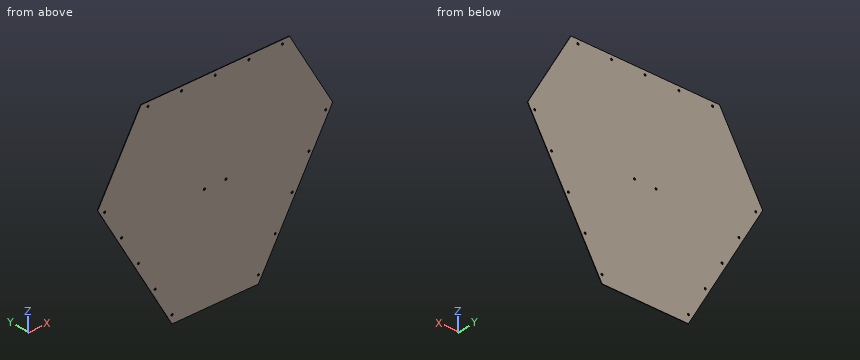
Autodesk Inventor part; units mm, degrees
ref_plane "YZ Plane" through (0, 0, 0) normal (1, 0, 0) x (0, 1, 0)
ref_plane "XZ Plane" through (0, 0, 0) normal (0, 1, 0) x (-1, 0, 0)
ref_plane "XY Plane" through (0, 0, 0) normal (0, 0, 1) x (1, 0, 0)
sketch "Sketch1" plane through (0, 0, 0) normal (0, 1, 0) x (-1, 0, 0)
  line L0 (101.5, -410.6115) -> (-101.7, -410.6115)
  line L1 (101.5, -410.6115) -> (406.3, 117.3176)
  line L2 (406.3, 117.3176) -> (304.7, 293.2939)
  line L3 (304.7, 293.2939) -> (-304.9, 293.2939)
  line L4 (-304.9, 293.2939) -> (-406.5, 117.3176)
  line L5 (-304.9, 293.2939) -> (-101.7, 293.2939) construction
  line L6 (-406.5, 117.3176) -> (-101.7, -410.6115)
  line L7 (-0.1, -410.6115) -> (-0.1, 293.2939) construction
  line L8 (-355.7, 205.3058) -> (253.9, -146.647) construction
  line L9 (-254.1, -146.647) -> (355.5, 205.3058) construction
  line L10 (34.1394, 19.7104) -> (0, 0) construction
  line L11 (0, 0) -> (-34.1644, -19.6671) construction
  line L12 (0, 0) -> (34.1144, -19.7537) construction
  circle A0 centre (-34.1644, -19.6671) radius 3.175 construction
  circle A1 centre (34.1144, -19.7537) radius 3.175 construction
  dimension "d0" = 120
  dimension "d1" = 203.2
  dimension "d3" = 609.6
  dimension "d8" = 203.2
  dimension "d10" = 120
  dimension "d13" = 609.6
  dimension "d15" = 203.2
  dimension "d16" = 120
  dimension "d17" = 609.6
  dimension "d18" = 120
  dimension "d22" = 101.6
  dimension "d122" = 39.4208
  dimension "d123" = 39.4208
  dimension "d124" = 6.35
  dimension "d125" = 6.35
extrude "Extrusion1" add sketch "Sketch1" against normal blind 1.5
sketch "Sketch2" plane through (0, 0, 0) normal (0, 1, 0) x (1, 0, 0)
  line L0 (-101.5, 410.6115) -> (101.7, 410.6115)
  line L1 (-406.3, -117.3176) -> (-101.5, 410.6115)
  line L2 (-304.7, -293.2939) -> (-406.3, -117.3176)
  line L3 (304.9, -293.2939) -> (-304.7, -293.2939)
  line L4 (406.5, -117.3176) -> (304.9, -293.2939)
  line L5 (101.7, 410.6115) -> (406.5, -117.3176)
  line L6 (0.1, 410.6115) -> (0.1, 350.0579) construction
  line L7 (0.1, 350.0579) -> (136.6606, 350.0579) construction
  line L8 (0.1, 350.0579) -> (-136.4606, 350.0579) construction
  line L9 (-355.5, -205.3058) -> (-303.059, -175.029) construction
  line L10 (355.7, -205.3058) -> (303.259, -175.029) construction
  line L11 (303.259, -175.029) -> (371.5394, -56.764) construction
  line L12 (303.259, -175.029) -> (234.9787, -293.2939) construction
  line L13 (-303.059, -175.029) -> (-234.7787, -293.2939) construction
  line L14 (-303.059, -175.029) -> (-371.3394, -56.764) construction
  line L15 (-371.3394, -56.764) -> (-234.7787, -293.2939)
  line L16 (-304.7, -293.2939) -> (-234.7787, -293.2939)
  line L17 (-304.7, -293.2939) -> (-406.3, -117.3176)
  line L18 (-371.3394, -56.764) -> (-406.3, -117.3176)
  line L19 (-101.5, 410.6115) -> (-136.4606, 350.0579)
  line L20 (-101.5, 410.6115) -> (101.7, 410.6115)
  line L21 (136.6606, 350.0579) -> (101.7, 410.6115)
  line L22 (136.6606, 350.0579) -> (-136.4606, 350.0579)
  line L23 (371.5394, -56.764) -> (234.9787, -293.2939)
  line L24 (304.9, -293.2939) -> (234.9787, -293.2939)
  line L25 (304.9, -293.2939) -> (406.5, -117.3176)
  line L26 (406.5, -117.3176) -> (371.5394, -56.764)
  point P0 (0, 0)
  dimension "d25" = 60.5536
  dimension "d26" = 60.5536
  dimension "d27" = 118.265
  dimension "d28" = 118.265
  dimension "d29" = 118.265
  dimension "d30" = 118.265
  dimension "d31" = 136.5606
  dimension "d32" = 136.5606
extrude "Extrusion2" cut sketch "Sketch2" against normal blind 25.4 contours L0 L5 L22 L1 | L15 L3 L2 L1 | L5 L4 L3 L23
sketch "Sketch5" plane through (0, -1.5, 0) normal (0, -1, 0) x (1, 0, 0)
  line L0 (-234.7787, 293.2939) -> (-371.3394, 56.764)
  line L1 (-136.4606, -350.0579) -> (136.6606, -350.0579)
  line L2 (136.6606, -350.0579) -> (371.5394, 56.764)
  line L3 (371.5394, 56.764) -> (234.9787, 293.2939)
  line L4 (-303.059, 175.029) -> (-281.062, 162.329) construction
  line L5 (303.259, 175.029) -> (281.262, 162.329) construction
  line L6 (0.1, -350.0579) -> (0.1, -324.6579) construction
  line L7 (-371.3394, 56.764) -> (-349.3423, 44.064) construction
  line L8 (234.9787, 293.2939) -> (212.9817, 280.5939) construction
  line L9 (371.5394, 56.764) -> (349.5423, 44.064) construction
  line L10 (-136.4606, -350.0579) -> (-136.4606, -324.6579) construction
  line L11 (136.6606, -350.0579) -> (136.6606, -324.6579) construction
  line L12 (-136.4606, -324.6579) -> (-136.4606, -324.6579) construction
  line L13 (136.6606, -324.6579) -> (136.6606, -324.6579) construction
  line L14 (-349.3423, 44.064) -> (-349.3423, 44.064) construction
  line L15 (-234.7787, 293.2939) -> (-212.7817, 280.5939) construction
  line L16 (-212.7817, 280.5939) -> (-212.7817, 280.5939) construction
  circle A0 centre (-349.3423, 44.064) radius 3.175
  circle A1 centre (-212.7817, 280.5939) radius 3.175
  circle A2 centre (212.9817, 280.5939) radius 3.175
  circle A3 centre (349.5423, 44.064) radius 3.175
  circle A4 centre (136.6606, -324.6579) radius 3.175
  circle A5 centre (-136.4606, -324.6579) radius 3.175
  line L17 (212.9817, 280.5939) -> (212.9817, 280.5939)
  line L18 (349.5423, 44.064) -> (349.5423, 44.064)
  line L19 (-212.7817, 280.5939) -> (-106.3408, 280.5939) construction
  line L20 (-106.3408, 280.5939) -> (0.1, 280.5939) construction
  line L21 (0.1, 280.5939) -> (106.5408, 280.5939) construction
  line L22 (106.5408, 280.5939) -> (212.9817, 280.5939) construction
  circle A6 centre (-106.3408, 280.5939) radius 3.175
  circle A7 centre (0.1, 280.5939) radius 3.175
  circle A8 centre (106.5408, 280.5939) radius 3.175
  line L23 (-349.3423, 44.064) -> (-296.1219, -48.1165) construction
  line L24 (-296.1219, -48.1165) -> (-242.9015, -140.297) construction
  line L25 (-242.9015, -140.297) -> (-189.6811, -232.4774) construction
  line L26 (-189.6811, -232.4774) -> (-136.4606, -324.6579) construction
  circle A9 centre (-296.1219, -48.1165) radius 3.175
  circle A10 centre (-242.9015, -140.297) radius 3.175
  circle A11 centre (-189.6811, -232.4774) radius 3.175
  line L27 (136.6606, -324.6579) -> (189.8811, -232.4774) construction
  line L28 (189.8811, -232.4774) -> (243.1015, -140.297) construction
  line L29 (243.1015, -140.297) -> (296.3219, -48.1165) construction
  line L30 (296.3219, -48.1165) -> (349.5423, 44.064) construction
  circle A12 centre (189.8811, -232.4774) radius 3.175
  circle A13 centre (243.1015, -140.297) radius 3.175
  circle A14 centre (296.3219, -48.1165) radius 3.175
  point P0 (0, 0)
  dimension "d67" = 25.4
  dimension "d68" = 25.4
  dimension "d69" = 25.4
  dimension "d70" = 25.4
  dimension "d71" = 25.4
  dimension "d72" = 25.4
  dimension "d73" = 0
  dimension "d74" = 0
  dimension "d75" = 0
  dimension "d76" = 0
  dimension "d77" = 6.35
  dimension "d78" = 6.35
  dimension "d79" = 6.35
  dimension "d80" = 6.35
  dimension "d81" = 6.35
  dimension "d82" = 6.35
  dimension "d83" = 0
  dimension "d84" = 0
  dimension "d87" = 425.7634
  dimension "d88" = 106.4408
  dimension "d89" = 106.4408
  dimension "d90" = 106.4408
  dimension "d91" = 106.4408
  dimension "d92" = 6.35
  dimension "d93" = 6.35
  dimension "d94" = 6.35
  dimension "d95" = 106.4408
  dimension "d96" = 106.4408
  dimension "d97" = 106.4408
  dimension "d98" = 106.4408
  dimension "d99" = 6.35
  dimension "d100" = 6.35
  dimension "d101" = 6.35
  dimension "d102" = 106.4408
  dimension "d103" = 106.4408
  dimension "d104" = 106.4408
  dimension "d105" = 106.4408
  dimension "d106" = 6.35
  dimension "d107" = 6.35
  dimension "d108" = 6.35
extrude "Extrusion5" cut sketch "Sketch5" against normal blind 25.4 contours A0 | A1 | A2 | A3 | A4 | A5
sketch "Sketch6" plane through (0, -1.5, 0) normal (0, -1, 0) x (1, 0, 0)
  circle A0 centre (-106.3408, 280.5939) radius 3.175
  circle A1 centre (0.1, 280.5939) radius 3.175
  circle A2 centre (106.5408, 280.5939) radius 3.175
  circle A3 centre (-296.1219, -48.1165) radius 3.175
  circle A4 centre (-242.9015, -140.297) radius 3.175
  circle A5 centre (-189.6811, -232.4774) radius 3.175
  circle A6 centre (189.8811, -232.4774) radius 3.175
  circle A7 centre (243.1015, -140.297) radius 3.175
  circle A8 centre (296.3219, -48.1165) radius 3.175
  point P0 (0, 0)
  dimension "d109" = 6.35
  dimension "d110" = 6.35
  dimension "d111" = 6.35
  dimension "d112" = 6.35
  dimension "d113" = 6.35
  dimension "d114" = 6.35
  dimension "d115" = 6.35
  dimension "d116" = 6.35
  dimension "d117" = 6.35
extrude "Extrusion6" cut sketch "Sketch6" against normal blind 25.4
sketch "Sketch7" plane through (0, -1.5, 0) normal (0, -1, 0) x (1, 0, 0)
  circle A0 centre (-34.1644, -19.6671) radius 3.175
  circle A1 centre (34.1144, -19.7537) radius 3.175
  point P0 (0, 0)
  dimension "d126" = 6.35
  dimension "d127" = 6.35
extrude "Extrusion7" cut sketch "Sketch7" against normal blind 25.4
equation "\"d8\" = d1"
equation "\"d13\" = d3"
equation "\"d15\" = d1"
equation "\"d124\" = d125"
equation "\"d88\" = 0.25 * d87"
equation "\"d90\" = d88"
equation "\"d91\" = d88"
equation "\"d92\" = d78"
equation "\"d93\" = d78"
equation "\"d94\" = d78"
equation "\"d95\" = d88"
equation "\"d96\" = d95"
equation "\"d97\" = d96"
equation "\"d98\" = d97"
equation "\"d99\" = d100"
equation "\"d100\" = d77"
equation "\"d101\" = d99"
equation "\"d102\" = d103"
equation "\"d103\" = d104"
equation "\"d104\" = d98"
equation "\"d105\" = d104"
equation "\"d106\" = d107"
equation "\"d107\" = d108"
equation "\"d108\" = d94"
equation "\"d109\" = d118"
equation "\"d110\" = d118"
equation "\"d111\" = d118"
equation "\"d112\" = d113"
equation "\"d113\" = d119"
equation "\"d114\" = d112"
equation "\"d115\" = d116"
equation "\"d116\" = d117"
equation "\"d117\" = d111"
equation "\"d126\" = d127"
properties part number "Base Plate" material "Prefabulated Amulite"
The model under review builds one solid part; all positions refer to its coordinate system, in mm. Coordinates: 2 decimals unless noted, no trailing zeros. Write each loop counter-clockwise with the first axis right and the second up, starting at its lowest first coordinate (ties: lowest second). Pieces come first, ordered by that corner, then holes. Notation, with made-up numbers: M 75.5,64 L 118.5,64 A18 cw 118.5,88 Z; hole C -27,52.5 d10. An arc over 180 degrees is marked long. Put each result on its own line as item: value.
1) Wall thickness on probe 1 along X at (y, z) = (-0.3, -288); probe 2 along X at (y, z) = (-1.35, -164.5); probe 3 along Z at (x, y) = (-208.5, -1.2): over which ranges is each line inside the solid? List them lowest first. Write a range as [from, to].
Computed:
probe 1: x = [-172.29, 172.49]
probe 2: x = [-243.59, 243.79]
probe 3: z = [-225.28, 293.29]
2) Clearance check with flat-ended pins moving along their axes: pin 1 Ø8.5 at (x, z) = (-136.46, -324.66) entering from +Y; pin 2 Ø4 at (x, z) = (189.88, -232.48) entering from -Y. State where each tip first meets the part, or that it passes through.
Computed:
pin 1: stops at y = 0
pin 2: passes through
3) Add section B-B on x = -280. Give the boundary of the cut face in (y, z).
Computed:
outline: M -1.5,-101.44 L 0,-101.44 L 0,214.97 L -1.5,214.97 Z
4) Add section A-A on y = -0.45. State how many separate pieces and enclosed holes the cut face has, then the cut area to 3 significant figures.
Computed:
separate pieces: 1
enclosed holes: 17
area: 350,000 mm2
5) Add section C-C on z = 153. Give the boundary of the cut face in (x, y), then the cut area to 3 significant figures.
Computed:
outline: M -315.78,-1.5 L 315.98,-1.5 L 315.98,0 L -315.78,0 Z
area: 948 mm2
